from build123d import *

# Parameters (mm, degrees)
SKETCH1_R           = 10
SKETCH1_R_2         = 9
BOSS_EXTRUDE1_DEPTH = 122
SKETCH3_R           = 2
CUT_EXTRUDE2_DEPTH  = 21


with BuildPart() as part:
    # Sketch1 → Boss-Extrude1 (new body)
    with BuildSketch(Plane(origin=(0, 0, 0), x_dir=(1, 0, 0), z_dir=(0, 1, 0))):
        Circle(SKETCH1_R)
        Circle(SKETCH1_R_2, mode=Mode.SUBTRACT)
    extrude(amount=BOSS_EXTRUDE1_DEPTH)

    # Sketch3 → Cut-Extrude2 (cut, through all)
    with BuildSketch(Plane.XY.offset(10)):
        with Locations((0, 109.5)):
            Circle(SKETCH3_R)
        with Locations((0, 12.5)):
            Circle(SKETCH3_R)
    extrude(amount=-CUT_EXTRUDE2_DEPTH, mode=Mode.SUBTRACT)


solid = part.part
Work out the finished part from the listing and answer in its coordinate system (mm). Coordinates: 2 decimals unless noted, no trailing zeros. Write each loop counter-clockwise with the first axis right and the second up, starting at its lowest first coordinate (ties: lowest second). Pieces come first, ordered by that corner, then holes.
1. For a pull along X with two mould halves and no side action, classify faces 1 (the cylindrical face through (-2.17, 60.15, 9.76)), 2 (the flat face through (-9, 0, -2)), 3 (the cylindrical face through (-1.172, 60.146, -8.923)) as +X half, -X half, draft (parallel to the pull), parting line (faces both ways), or undercut.
Results list:
face 1: parting line
face 2: draft
face 3: undercut
2. The part is cut by section B-B, the plane x = 0. Write down the section's boundary in (y, z), and give its area (3 significant figures).
Results list:
outline: (0, -10) - (10.5, -10) - (10.5, -9) - (0, -9) - close; (0, 9) - (10.5, 9) - (10.5, 10) - (0, 10) - close; (14.5, -10) - (107.5, -10) - (107.5, -9) - (14.5, -9) - close; (14.5, 9) - (107.5, 9) - (107.5, 10) - (14.5, 10) - close; (111.5, -10) - (122, -10) - (122, -9) - (111.5, -9) - close; (111.5, 9) - (122, 9) - (122, 10) - (111.5, 10) - close
area: 228 mm2
3. The part is cut by section A-A, the plane z = 0. Write down the section's boundary in (x, y), and give its area (3 significant figures).
Results list:
outline: (-10, 0) - (-9, 0) - (-9, 122) - (-10, 122) - close; (9, 0) - (10, 0) - (10, 122) - (9, 122) - close
area: 244 mm2
4. Flat-ended cylindrical pins translate along their axes: pin 1 (4 mm diameter, centred on x = 6.5, z = -2, fed in from -Y); pin 2 (8 mm diameter, centred on x = 7.5, y = 103.5, fed in from +Z); pin 3 (1.5 mm diameter, centred on x = 7, y = 67, fed in from +Z); pin 4 (2 mm diameter, centred on y = 45.5, z = 7.5, fed in from -X). Find the tip coordinate at first contact, or state that the pin passes through.
Results list:
pin 1: passes through
pin 2: stops at z = 9.37
pin 3: stops at z = 7.81
pin 4: stops at x = -7.6
5. The part is cut by section D-D, the plane y = 74. Write down the section's boundary in (x, z), and give its area (3 significant figures).
Results list:
outline: circle Ø20 at (0, 0); hole circle Ø18 at (0, 0)
area: 59.7 mm2
6. The part is cut by section C-C, the plane x = -7.5. Write down the section's boundary in (y, z).
Results list:
outline: (0, -6.61) - (122, -6.61) - (122, -4.97) - (0, -4.97) - close; (0, 4.97) - (122, 4.97) - (122, 6.61) - (0, 6.61) - close
7. Consider line 1 along Y through (x, z) = (0, -9.55); line 2 along X through (y, z) = (88, -0.25); line 3 along Z through (x, y) = (-1, 6). Determine where each line is inside the solid, lowest interval first.
Results list:
line 1: y = 0 to 10.5, 14.5 to 107.5, 111.5 to 122
line 2: x = -10 to -9, 9 to 10
line 3: z = -9.95 to -8.94, 8.94 to 9.95
